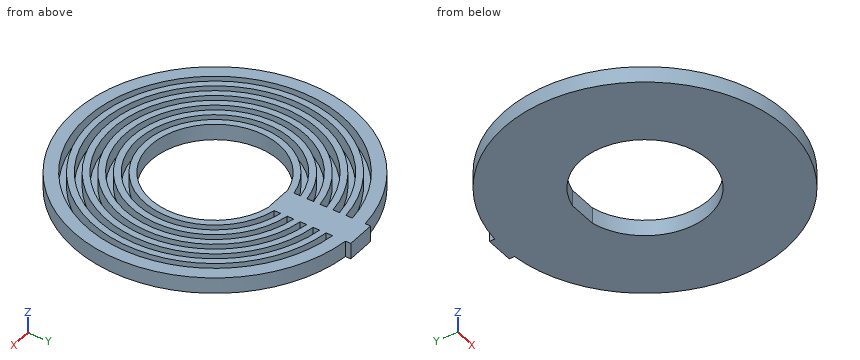
```python
from build123d import *

# Parameters (mm, degrees)
CROQUIS1_R              = 22
CROQUIS1_R_2            = 10
SALIENTE_EXTRUIR1_DEPTH = 2.5
CROQUIS2_R              = 20
CROQUIS2_R_2            = 19
CROQUIS2_R_3            = 18
CROQUIS2_R_4            = 17
CROQUIS2_R_5            = 16
CROQUIS2_R_6            = 15
CROQUIS2_R_7            = 14
CROQUIS2_R_8            = 13
CROQUIS2_R_9            = 12
CROQUIS2_R_10           = 11
CORTAR_EXTRUIR1_DEPTH   = 2.25
SALIENTE_EXTRUIR2_DEPTH = 2.5


with BuildPart() as part:
    # Croquis1 → Saliente-Extruir1 (new body)
    with BuildSketch(Plane.XY):
        Circle(CROQUIS1_R)
        Circle(CROQUIS1_R_2, mode=Mode.SUBTRACT)
    extrude(amount=SALIENTE_EXTRUIR1_DEPTH)

    # Croquis2 → Cortar-Extruir1 (cut)
    # profile 1 of 5: a face of its own
    with BuildSketch(Plane.XY.offset(2.5)):
        Circle(CROQUIS2_R)
        Circle(CROQUIS2_R_2, mode=Mode.SUBTRACT)
    # profile 2 of 5: a face of its own
    with BuildSketch(Plane.XY.offset(2.5)):
        Circle(CROQUIS2_R_3)
        Circle(CROQUIS2_R_4, mode=Mode.SUBTRACT)
    # profile 3 of 5: a face of its own
    with BuildSketch(Plane.XY.offset(2.5)):
        Circle(CROQUIS2_R_5)
        Circle(CROQUIS2_R_6, mode=Mode.SUBTRACT)
    # profile 4 of 5: a face of its own
    with BuildSketch(Plane.XY.offset(2.5)):
        Circle(CROQUIS2_R_7)
        Circle(CROQUIS2_R_8, mode=Mode.SUBTRACT)
    # profile 5 of 5: a face of its own
    with BuildSketch(Plane.XY.offset(2.5)):
        Circle(CROQUIS2_R_9)
        Circle(CROQUIS2_R_10, mode=Mode.SUBTRACT)
    extrude(amount=-CORTAR_EXTRUIR1_DEPTH, mode=Mode.SUBTRACT)

    # Croquis3 → Saliente-Extruir2 (add)
    with BuildSketch(Plane.XY.offset(2.5)):
        with BuildLine():
            ThreePointArc((2.222048604, 9.75), (0, 10), (-2.222048604, 9.75))
            Line((-2.222048604, 9.75), (2.222048604, 9.75))
        make_face()
        with BuildLine():
            ThreePointArc((-2.222048604, 10.773230713), (0, 11), (2.222048604, 10.773230713))
            Line((2.222048604, 10.773230713), (2.222048604, 11.792476415))
            ThreePointArc((2.222048604, 11.792476415), (0, 12), (-2.222048604, 11.792476415))
            Line((-2.222048604, 11.792476415), (-2.222048604, 10.773230713))
        make_face()
        with BuildLine():
            ThreePointArc((-2.222048604, 12.808688457), (0, 13), (2.222048604, 12.808688457))
            Line((2.222048604, 12.808688457), (2.222048604, 13.822535947))
            ThreePointArc((2.222048604, 13.822535947), (0, 14), (-2.222048604, 13.822535947))
            Line((-2.222048604, 13.822535947), (-2.222048604, 12.808688457))
        make_face()
        with BuildLine():
            ThreePointArc((-2.222048604, 14.834503699), (0, 15), (2.222048604, 14.834503699))
            Line((2.222048604, 14.834503699), (2.222048604, 15.844951877))
            ThreePointArc((2.222048604, 15.844951877), (0, 16), (-2.222048604, 15.844951877))
            Line((-2.222048604, 15.844951877), (-2.222048604, 14.834503699))
        make_face()
        with BuildLine():
            ThreePointArc((-2.222048604, 16.854153791), (0, 17), (2.222048604, 16.854153791))
            Line((2.222048604, 16.854153791), (2.222048604, 17.862320678))
            ThreePointArc((2.222048604, 17.862320678), (0, 18), (-2.222048604, 17.862320678))
            Line((-2.222048604, 17.862320678), (-2.222048604, 16.854153791))
        make_face()
        with BuildLine():
            ThreePointArc((-2.222048604, 18.869618438), (0, 19), (2.222048604, 18.869618438))
            Line((2.222048604, 18.869618438), (2.222048604, 19.87617921))
            ThreePointArc((2.222048604, 19.87617921), (0, 20), (-2.222048604, 19.87617921))
            Line((-2.222048604, 19.87617921), (-2.222048604, 18.869618438))
        make_face()
        with BuildLine():
            ThreePointArc((-2.222048604, 21.887496431), (0, 22), (2.222048604, 21.887496431))
            Line((2.222048604, 21.887496431), (2.222048604, 22.721977181))
            Line((2.222048604, 22.721977181), (-2.222048604, 22.721977181))
            Line((-2.222048604, 22.721977181), (-2.222048604, 21.887496431))
        make_face()
    extrude(amount=-SALIENTE_EXTRUIR2_DEPTH)


solid = part.part
```
Geometry: final body of the model. Coordinates: model frame, mm. Round coordinates to 2 decimals unless told otherwise and drop trailing zeros. Order: outer loops, then holes, each group sorted by start corner. A loop starts at its lowest first (then second) coordinate and runs counter-clockwise, first axis right, second up. Notation, with made-up numbers: M 7.25,23.5 L 18.25,23.5 A21 ccw 18.25,27.5 Z; hole C 51,-31 d5. An arc over 180 degrees is marked long. Use one line per item in the form item = value. Start each with the question number.
Q1. Pin query (flat end, axial travel): pin 1 Ø0.5 at (y, z) = (11.5, 1) entering from -X; pin 2 Ø0.8 at (y, z) = (13.5, 1.5) entering from -X; pin 3 Ø0.5 at (y, z) = (19.5, 1) entering from +X. Return the tip coordinate at first contact, or that it passes through.
Q2. Material intervals for line 1 (X direction, y = -8.5, z = 0.2); line 2 (Z direction, x = 11, y = -8); line 3 (X direction, y = 20, z = 0.1), sorted ascending. Write a range as [from, to].
Q3. Cut plane B-B (x = 0). Return loops of the section in (y, z).
Q4. Cut plane A-A (z = 2). Return loops of the section in (x, y).
Geometry results:
q1.pin_1 = -18.91
q1.pin_2 = -17.67
q1.pin_3 = 10.65
q2.line_1 = [-20.29, -5.27], [5.27, 20.29]
q2.line_2 = [0, 0.25]
q2.line_3 = [-9.17, 9.17]
q3.outline = M -22,0 L -10,0 L -10,2.5 L -11,2.5 L -11,0.25 L -12,0.25 L -12,2.5 L -13,2.5 L -13,0.25 L -14,0.25 L -14,2.5 L -15,2.5 L -15,0.25 L -16,0.25 L -16,2.5 L -17,2.5 L -17,0.25 L -18,0.25 L -18,2.5 L -19,2.5 L -19,0.25 L -20,0.25 L -20,2.5 L -22,2.5 Z; M 9.75,0 L 22.72,0 L 22.72,2.5 L 9.75,2.5 Z
q4.outline = M -2.22,21.89 A22 ccw long 2.22,21.89 L 2.22,22.72 L -2.22,22.72 Z; hole M -2.22,9.75 A10 ccw long 2.22,9.75 Z; hole M -2.22,10.77 L -2.22,11.79 A12 ccw long 2.22,11.79 L 2.22,10.77 A11 cw long Z; hole M -2.22,12.81 L -2.22,13.82 A14 ccw long 2.22,13.82 L 2.22,12.81 A13 cw long Z; hole M -2.22,14.83 L -2.22,15.84 A16 ccw long 2.22,15.84 L 2.22,14.83 A15 cw long Z; hole M -2.22,16.85 L -2.22,17.86 A18 ccw long 2.22,17.86 L 2.22,16.85 A17 cw long Z; hole M -2.22,18.87 L -2.22,19.88 A20 ccw long 2.22,19.88 L 2.22,18.87 A19 cw long Z
